```python
from build123d import *

# Parameters (mm, degrees)
BOSS_EXTRUDE1_DEPTH = 10.5
SKETCH2_R           = 14.75
BOSS_EXTRUDE2_DEPTH = 14
SKETCH3_R           = 13
BOSS_EXTRUDE3_DEPTH = 14
BOSS_EXTRUDE4_DEPTH = 16
SKETCH5_R           = 10.75
BOSS_EXTRUDE5_DEPTH = 20
SKETCH6_R           = 2.1
BOSS_EXTRUDE6_DEPTH = 2.5
CUT_EXTRUDE1_REACH  = 63.722
SKETCH7_R           = 7.5
SKETCH8_R           = 12.5
SKETCH8_R_2         = 10.75
BOSS_EXTRUDE7_DEPTH = 2
BOSS_EXTRUDE8_DEPTH = 15


with BuildPart() as part:
    # Sketch1 → Boss-Extrude1 (new body)
    with BuildSketch(Plane.YZ):
        Polygon((0, 12.413030788), (-10.75, 6.206515394), (-10.75, -6.206515394), (0, -12.413030788), (10.75, -6.206515394), (10.75, 6.206515394), align=None)
    extrude(amount=BOSS_EXTRUDE1_DEPTH)

    # Sketch2 → Boss-Extrude2 (add)
    with BuildSketch(Plane.YZ.offset(10.5)):
        with Locations(Location((0, 0, 0), (0, 0, 270))):
            Circle(SKETCH2_R)
    extrude(amount=BOSS_EXTRUDE2_DEPTH)

    # Sketch3 → Boss-Extrude3 (add)
    with BuildSketch(Plane.YZ.offset(24.5)):
        with Locations(Location((0, 0, 0), (0, 0, 270))):
            Circle(SKETCH3_R)
    extrude(amount=BOSS_EXTRUDE3_DEPTH)

    # Sketch4 → Boss-Extrude4 (add)
    with BuildSketch(Plane.YZ.offset(38.5)):
        Polygon((0, 12.413030788), (-10.75, 6.206515394), (-10.75, -6.206515394), (0, -12.413030788), (10.75, -6.206515394), (10.75, 6.206515394), align=None)
    extrude(amount=BOSS_EXTRUDE4_DEPTH)

    # Sketch5 → Boss-Extrude5 (add)
    with BuildSketch(Plane(origin=(0, 0, 0), x_dir=(0, 1, 0), z_dir=(0, 0, 1))):
        with Locations(Location((0, -27.25, 0), (0, 0, 14.821821062))):
            Circle(SKETCH5_R)
    extrude(amount=BOSS_EXTRUDE5_DEPTH)

    # Sketch6 → Boss-Extrude6 (add)
    with BuildSketch(Plane.XY.offset(20)):
        with BuildLine():
            Line((13, -18.25), (41.5, -18.25))
            ThreePointArc((41.5, -18.25), (44.328427125, -17.078427125), (45.5, -14.25))
            Line((45.5, -14.25), (45.5, 14.25))
            ThreePointArc((45.5, 14.25), (44.328427125, 17.078427125), (41.5, 18.25))
            Line((41.5, 18.25), (13, 18.25))
            ThreePointArc((13, 18.25), (10.171572875, 17.078427125), (9, 14.25))
            Line((9, 14.25), (9, -14.25))
            ThreePointArc((9, -14.25), (10.171572875, -17.078427125), (13, -18.25))
        make_face()
        with Locations((14.25, 13)):
            Circle(SKETCH6_R, mode=Mode.SUBTRACT)
        with Locations((40.25, 13)):
            Circle(SKETCH6_R, mode=Mode.SUBTRACT)
        with Locations((40.25, -13)):
            Circle(SKETCH6_R, mode=Mode.SUBTRACT)
        with Locations((14.25, -13)):
            Circle(SKETCH6_R, mode=Mode.SUBTRACT)
    extrude(amount=BOSS_EXTRUDE6_DEPTH)

    # Sketch7 → Cut-Extrude1 (cut, up to next)
    with BuildSketch(Plane.YZ.offset(54.5), mode=Mode.PRIVATE) as cut_extrude1_sk1:
        with Locations(Location((0, 0, 0), (0, 0, 270))):
            Circle(SKETCH7_R)
    cut_extrude1_tool1 = extrude(cut_extrude1_sk1.sketch, amount=-CUT_EXTRUDE1_REACH, mode=Mode.PRIVATE) & part.part
    add(cut_extrude1_tool1.solids().sort_by_distance((54.5, 0, 0))[0], mode=Mode.SUBTRACT)

    # Sketch8 → Boss-Extrude7 (add)
    with BuildSketch(Plane.XY.offset(22.5)):
        with Locations(Location((27.25, 0, 0), (0, 0, 180))):
            Circle(SKETCH8_R)
        with Locations(Location((27.25, 0, 0), (0, 0, 104.821821062))):
            Circle(SKETCH8_R_2, mode=Mode.SUBTRACT)
    extrude(amount=BOSS_EXTRUDE7_DEPTH)

    # Sketch9 → Boss-Extrude8 (add)
    with BuildSketch(Plane.XY.offset(22.5)):
        with BuildLine():
            Line((23.815251101, -2.05), (30.684748899, -2.05))
            ThreePointArc((30.684748899, -2.05), (31.25, 0), (30.684748899, 2.05))
            Line((30.684748899, 2.05), (23.815251101, 2.05))
            ThreePointArc((23.815251101, 2.05), (23.25, 0), (23.815251101, -2.05))
        make_face()
    extrude(amount=BOSS_EXTRUDE8_DEPTH)


solid = part.part
```
For this review, take the finished solid that the model builds, in its own axes (mm). A direction names the side the tool comes from. Give positions to 0.01 mm unless a question says otherwise; leave off trailing zeros. Write each loop counter-clockwise with the first axis right and the second up, starting at its lowest first coordinate (ties: lowest second). Pieces come first, ordered by that corner, then holes.
Item 1: The part is to be moulded in two halves that separate along X. For faces 1 (the face through (38.15, 13.09, 21.23)), 2 (the face through (9, 0, 21)), 3 (the face through (27, 0, 37.5)), 4 (the face through (54.5, -7.3, -2.6)), say which applies: +X half, -X half, draft (parallel to the pull), parting line (faces both ways), or undercut.
Item 2: Machinability: for faces 5 (the face through (46.388, 5.45, 9.266)), 6 (the face through (46, -10.75, 0)), 7 (the face through (17.4, 4.43, -14.07)), 8 (the face through (5.176, -5.45, -9.266)), which of the approach directions +Z, -Z, +X, -X, +Y, -Y give a long, thin tool a straight path to every point of the face, cutting with its end or side? Answer none if there is none.
Item 3: Insertion check: P1, Ø6, axis at x = 37.5, z = 2, coming from the -Y side; P2, Ø5.5, axis at x = 28, z = 31, coming from the -Y side; P3, Ø5.5, axis at x = 29, z = 33.5, coming from the +Y side; P4, Ø11, axis at x = 19, y = 5, coming from the -Z side. Each pin has a flat end and moves straight along its axis. Give the tip position at first contact, or say it passes through.
Item 4: Take a section at A-A (z = 0). Give the boundary of the cut face in (x, y).
Item 5: Take a section at D-D (x = 36). Give the boundary of the cut face in (y, z) (3 decimals).
Item 6: Wall thickness on probe 1 along Y at (x, z) = (27, 23); probe 2 along Y at (x, z) = (14.25, 20.5); probe 3 along Y at (x, z) = (29.5, 26.5): over which ranges is each line inside the solid? List them lowest first.
Item 7: Take a section at B-B (x = 27.25). Give the boundary of the cut face in (y, z), and give its area (3 significant figures).
Established:
1. face 1: undercut
1. face 2: -X half
1. face 3: draft
1. face 4: +X half
2. face 5: +X, +Y
2. face 6: -Z, +X, -Y
2. face 7: -X
2. face 8: -Z, -X, -Y
3. P1: stops at y = -13
3. P2: stops at y = -2.05
3. P3: stops at y = 2.05
3. P4: stops at z = -14.75
4. outline: (0, -10.75) - (10.5, -10.75) - (10.5, -14.75) - (24.5, -14.75) - (24.5, -13) - (38.5, -13) - (38.5, -10.75) - (54.5, -10.75) - (54.5, -7.5) - (0, -7.5) - close; (0, 7.5) - (54.5, 7.5) - (54.5, 10.75) - (38.5, 10.75) - (38.5, 13) - (24.5, 13) - (24.5, 14.75) - (10.5, 14.75) - (10.5, 10.75) - (0, 10.75) - close
5. outline: (-18.25, 20) - (-6.245, 20) - (-6.245, 11.402) arc R13 ccw (long way) to (6.245, 11.402) - (6.245, 20) - (18.25, 20) - (18.25, 22.5) - (8.927, 22.5) - (8.927, 24.5) - (6.245, 24.5) - (6.245, 22.5) - (-6.245, 22.5) - (-6.245, 24.5) - (-8.927, 24.5) - (-8.927, 22.5) - (-18.25, 22.5) - close; hole circle Ø15 at (0, 0)
6. probe 1: y = -12.5 to -10.75, -2.05 to 2.05, 10.75 to 12.5
6. probe 2: y = -18.25 to -15.1, -10.9 to 10.9, 15.1 to 18.25
6. probe 3: y = -2.05 to 2.05
7. outline: (-18.25, 20) - (-10.75, 20) - (-10.75, 7.31) arc R13 ccw (long way) to (10.75, 7.31) - (10.75, 20) - (18.25, 20) - (18.25, 22.5) - (12.5, 22.5) - (12.5, 24.5) - (10.75, 24.5) - (10.75, 22.5) - (2.05, 22.5) - (2.05, 37.5) - (-2.05, 37.5) - (-2.05, 22.5) - (-10.75, 22.5) - (-10.75, 24.5) - (-12.5, 24.5) - (-12.5, 22.5) - (-18.25, 22.5) - close; hole circle Ø15 at (0, 0)
7. area: 701 mm2
